The listing builds one solid part. Answer for the finished solid, in the listing's coordinates (mm). Face numbers are marked on the shaded views. Give positions to 0.01 mm unless a question says otherwise; leave off trailing zeros. Loops run counter-clockwise (first coordinate to the right, second up) from the corner with the lowest first, then second, coordinate; pieces in that order, holes last. Notation, with made-up numbers: (38.25, 73) - (68.25, 73) arc R27 cw to (68.25, 106) - close; hole circle Ø2 at (-19, 16.5). An arc over 180 degrees is marked (long way). Write each question's results on one line, items separated by ' | '.
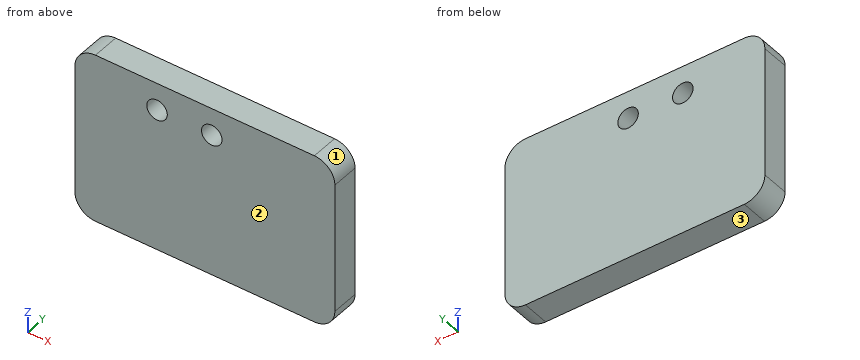
from build123d import *

# Parameters (mm, degrees)
SKETCH_1_W      = 38
SKETCH_1_H      = 25
SKETCH_1_R      = 1.5
EXTRUDE_1_DEPTH = 4
FILLET_1_R      = 3


with BuildPart() as part:
    # 草图1 → 凸台-拉伸1 (new body)
    with BuildSketch(Plane(origin=(0, 0, 0), x_dir=(1, 0, 0), z_dir=(0, 1, 0))):
        Rectangle(SKETCH_1_W, SKETCH_1_H)
        with Locations(Location((-7, -8.5, 0), (0, 0, 270))):
            Circle(SKETCH_1_R, mode=Mode.SUBTRACT)
        with Locations(Location((1, -8.5, 0), (0, 0, 270))):
            Circle(SKETCH_1_R, mode=Mode.SUBTRACT)
    extrude(amount=EXTRUDE_1_DEPTH)

    # 圆角1
    fillet_1_edges = [part.edges().sort_by_distance(p)[0] for p in [
        (-19, 2, 12.5),
        (-19, 2, -12.5),
        (19, 2, -12.5),
        (19, 2, 12.5),
    ]]
    fillet(fillet_1_edges, radius=FILLET_1_R)


solid = part.part
Item 1: Find the intervals of material crossed by line 1 along X through (y, z) = (1, 8.5); line 2 along Z through (x, y) = (-6.5, 0.6); line 3 along Z through (x, y) = (-17, 1.15), in increasing order. Write a range as [from, to].
Values found:
line 1: x = [-19, -8.5], [-5.5, -0.5], [2.5, 19] | line 2: z = [-12.5, 7.09], [9.91, 12.5] | line 3: z = [-12.33, 12.33]
Item 2: A cutting plane is placed at A-A, the plane x = 1. Determine the outline of the cut face in (y, z).
Values found:
outline: (0, -12.5) - (4, -12.5) - (4, 7) - (0, 7) - close; (0, 10) - (4, 10) - (4, 12.5) - (0, 12.5) - close
Item 3: A cutting plane is placed at C-C, the plane z = 8.5. Determine the outline of the cut face in (x, y).
Values found:
outline: (-19, 0) - (-8.5, 0) - (-8.5, 4) - (-19, 4) - close; (-5.5, 0) - (-0.5, 0) - (-0.5, 4) - (-5.5, 4) - close; (2.5, 0) - (19, 0) - (19, 4) - (2.5, 4) - close
Item 4: A flat-ended cylindrical pin translates along its axis: P1, Ø2.5, axis at x = -7, z = 8.5, coming from the +Y side. Find the tip coordinate at first contact, or state that the pin passes through.
Values found:
P1: passes through
Item 5: A cutting plane is placed at D-D, the plane x = -6.5. Determine the outline of the cut face in (y, z), plus the area to 3 significant figures.
Values found:
outline: (0, -12.5) - (4, -12.5) - (4, 7.09) - (0, 7.09) - close; (0, 9.91) - (4, 9.91) - (4, 12.5) - (0, 12.5) - close | area: 88.7 mm²
Item 6: For a pull along Z with two mould halves and no side action, classify the marked faces 1, 2 and 3 as released by +Z, released by -Z, zero draft, split by the parting line, or undercut.
Values found:
face 1: released by +Z | face 2: zero draft | face 3: released by -Z
Item 7: A cutting plane is placed at B-B, the plane y = 1.85. Determine the outline of the cut face in (x, z), plus the area to 3 significant figures.
Values found:
outline: (-19, -9.5) arc R3 ccw to (-16, -12.5) - (16, -12.5) arc R3 ccw to (19, -9.5) - (19, 9.5) arc R3 ccw to (16, 12.5) - (-16, 12.5) arc R3 ccw to (-19, 9.5) - close; hole circle Ø3 at (-7, 8.5); hole circle Ø3 at (1, 8.5) | area: 928 mm²
